```python
from build123d import *

# Parameters (mm, degrees)
SKETCH_W        = 84
SKETCH_H        = 140
PAD_DEPTH       = 40
SKETCH001_W     = 80
SKETCH001_H     = 136
POCKET_DEPTH    = 36
SKETCH004_W     = 80
SKETCH004_H     = 115
POCKET003_DEPTH = 4
SKETCH005_W     = 79.75218
SKETCH005_H     = 36
POCKET004_DEPTH = 2
SKETCH006_W     = 80
SKETCH006_H     = 115
POCKET005_DEPTH = 2


with BuildPart() as part:
    # Sketch → Pad (new body)
    with BuildSketch(Plane.XY):
        Rectangle(SKETCH_W, SKETCH_H)
    extrude(amount=PAD_DEPTH)

    # Sketch001 → Pocket (cut)
    with BuildSketch(Plane.XY.offset(38)):
        Rectangle(SKETCH001_W, SKETCH001_H)
    extrude(amount=-POCKET_DEPTH, mode=Mode.SUBTRACT)

    # Sketch004 → Pocket003 (cut)
    with BuildSketch(Plane.XY):
        with Locations((0, 0.5)):
            Rectangle(SKETCH004_W, SKETCH004_H)
    extrude(amount=POCKET003_DEPTH, mode=Mode.SUBTRACT)

    # Sketch005 → Pocket004 (cut)
    with BuildSketch(Plane.XZ.offset(-70)):
        with Locations((0.12391, 20)):
            Rectangle(SKETCH005_W, SKETCH005_H)
    extrude(amount=POCKET004_DEPTH, mode=Mode.SUBTRACT)

    # Sketch006 → Pocket005 (cut)
    with BuildSketch(Plane.XY.offset(40)):
        with Locations((0, 0.5)):
            Rectangle(SKETCH006_W, SKETCH006_H)
    extrude(amount=-POCKET005_DEPTH, mode=Mode.SUBTRACT)


solid = part.part
```
Model file for the job. Use its own axes, mm. A direction names the side the tool comes from. Coordinates: 2 decimals unless noted, no trailing zeros. Write each loop counter-clockwise with the first axis right and the second up, starting at its lowest first coordinate (ties: lowest second). Pieces come first, ordered by that corner, then holes. Notation, with made-up numbers: (71, -40) - (81, -40) arc R23 ccw to (81, -5) - close; hole circle Ø6 at (15.5, 87.5). An arc over 180 degrees is marked (long way). Use a Markdown table: item, result. Add a question column.
Item 1: Drill centre lines: line 1 along X through (y, z) = (49.5, 36.5); line 2 along Z through (x, y) = (33, -61.5); line 3 along Y through (x, z) = (26, 29.5). Where is each one in solid material? Low to high.
Item 2: Band-saw the part on C-C, the plane z = 32. Write the cut outline in (x, y).
Item 3: Drop a flat-ended pin along its axis: pin 1 (1.5 mm diameter, centred on x = -24.5, z = 33, fed in from +Y). Give the stop position or say it passes through.
Item 4: Band-saw the part on D-D, the plane y = 60.5. Write the cut outline in (x, z), and give its area (3 significant figures).
Item 5: Band-saw the part on B-B, the plane y = 25.5. Write the cut outline in (x, z), and give its area (3 significant figures).
Item 6: 3-axis set-ups, long thin cutter, end or side, ignore diameter. For faces 1 (the face through (-40, -1, 20)), 2 (the face through (-1, -62, 2)), 3 (the face through (-1, -70, 20)): which of +Z, -Z, +X, -X, +Y, -Y reach the whole face in a straight line?
Item 7: Band-saw the part on A-A, the plane x = 14. Write the cut outline in (y, z).
Item 8: Two-plate mould, pull along X, no slides. Class faces 4 (the face through (-42, -1, 20)), 5 (the face through (-41, -5, 40)), 6 (the face through (42, -1, 20)), 7 (the face through (-1, -62, 38)): pulls with the +X half, pulls with the -X half, needs draft (parallel to the pull), parting line crosses it, or undercut.
A:
| question | item | result |
|---|---|---|
| 1 | line 1 | x = -42 to -40, 40 to 42 |
| 1 | line 2 | z = 0 to 2, 38 to 40 |
| 1 | line 3 | y = -70 to -68 |
| 2 | outline | (-42, -70) - (42, -70) - (42, 70) - (40, 70) - (40, -68) - (-40, -68) - (-40, 68) - (-39.75, 68) - (-39.75, 70) - (-42, 70) - close |
| 3 | pin 1 | stops at y = -68 |
| 4 | outline | (-42, 0) - (42, 0) - (42, 40) - (-42, 40) - close; hole (-40, 2) - (40, 2) - (40, 38) - (-40, 38) - close |
| 4 | area | 480 mm² |
| 5 | outline | (-42, 0) - (-40, 0) - (-40, 40) - (-42, 40) - close; (40, 0) - (42, 0) - (42, 40) - (40, 40) - close |
| 5 | area | 160 mm² |
| 6 | face 1 | none |
| 6 | face 2 | +Y |
| 6 | face 3 | +Z, -Z, +X, -X, -Y |
| 7 | outline | (-70, 0) - (-57, 0) - (-57, 2) - (-68, 2) - (-68, 38) - (-57, 38) - (-57, 40) - (-70, 40) - close; (58, 0) - (70, 0) - (70, 2) - (58, 2) - close; (58, 38) - (70, 38) - (70, 40) - (58, 40) - close |
| 8 | face 4 | pulls with the -X half |
| 8 | face 5 | needs draft |
| 8 | face 6 | pulls with the +X half |
| 8 | face 7 | undercut |
